from build123d import *

# Parameters (mm, degrees)
DELETE_START           = -13.5
DELETE_FACE_1_DEPTH    = 27
MOVE_FACE_1_BY         = 7
MOVE_FACE_2_BY         = 5.5
SKETCH_2_W             = 48.263019836
SKETCH_2_H             = 43.058184364
CUT_EXTRUDE_1_DEPTH    = 20
EXTRUDE_1_DEPTH        = 2
EXTRUDE_1_DEPTH_BACK   = 5
SKETCH_3_W             = 20
SKETCH_3_H             = 19
HOLE_WIZARD_M5_1_D     = 4.2
HOLE_WIZARD_M5_1_DEPTH = 20
HOLE_WIZARD_M5_1_TIP   = 1.2618073


with BuildPart() as part:
    # Delete Face 1: read off the stored shape, not the designer's step
    # Delete Face 1 outline → Delete Face 1 (new body)
    with BuildSketch(Plane.YZ.offset(DELETE_START)):
        with BuildLine():
            ThreePointArc((-8.364285714, 23.895568572), (-8.397831007, 23.931741933), (-8.41, 23.979551078))
            Line((-8.41, 23.979551078), (-8.41, 26.020448922))
            ThreePointArc((-8.41, 26.020448922), (-8.397831007, 26.068258067), (-8.364285714, 26.104431428))
            ThreePointArc((-8.364285714, 26.104431428), (-7.725958169, 26.423724028), (-7.033327746, 26.595982314))
            ThreePointArc((-7.033327746, 26.595982314), (-6.723611818, 26.762379014), (-6.6, 27.091517187))
            Line((-6.6, 27.091517187), (-6.6, 27.908482813))
            ThreePointArc((-6.6, 27.908482813), (-6.723615527, 28.237625227), (-7.033338915, 28.404019189))
            ThreePointArc((-7.033338915, 28.404019189), (-7.725963455, 28.576277924), (-8.364285714, 28.895568572))
            ThreePointArc((-8.364285714, 28.895568572), (-8.397831007, 28.931741933), (-8.41, 28.979551078))
            Line((-8.41, 28.979551078), (-8.41, 31.020448922))
            ThreePointArc((-8.41, 31.020448922), (-8.397831007, 31.068258067), (-8.364285714, 31.104431428))
            ThreePointArc((-8.364285714, 31.104431428), (-7.725958168, 31.423724029), (-7.033327744, 31.595982314))
            ThreePointArc((-7.033327744, 31.595982314), (-6.723611817, 31.762379015), (-6.6, 32.091517187))
            Line((-6.6, 32.091517187), (-6.6, 32.908482813))
            ThreePointArc((-6.6, 32.908482813), (-6.602116164, 32.954435895), (-6.608446743, 33))
            Line((-6.608446743, 33), (-12.6, 33))
            Line((-12.6, 33), (-12.6, -33))
            Line((-12.6, -33), (-6.608446743, -33))
            ThreePointArc((-6.608446743, -33), (-6.602116164, -32.954435895), (-6.6, -32.908482813))
            Line((-6.6, -32.908482813), (-6.6, -32.091517187))
            ThreePointArc((-6.6, -32.091517187), (-6.723615531, -31.762374768), (-7.033338927, -31.595980809))
            ThreePointArc((-7.033338927, -31.595980809), (-7.72596346, -31.423722074), (-8.364285714, -31.104431428))
            ThreePointArc((-8.364285714, -31.104431428), (-8.397831007, -31.068258067), (-8.41, -31.020448922))
            Line((-8.41, -31.020448922), (-8.41, -28.979551078))
            ThreePointArc((-8.41, -28.979551078), (-8.397831007, -28.931741933), (-8.364285714, -28.895568572))
            ThreePointArc((-8.364285714, -28.895568572), (-7.725958168, -28.576275971), (-7.033327744, -28.404017686))
            ThreePointArc((-7.033327744, -28.404017686), (-6.723611817, -28.237620985), (-6.6, -27.908482813))
            Line((-6.6, -27.908482813), (-6.6, -27.091517187))
            ThreePointArc((-6.6, -27.091517187), (-6.723615528, -26.762374772), (-7.033338917, -26.595980811))
            ThreePointArc((-7.033338917, -26.595980811), (-7.725963456, -26.423722076), (-8.364285714, -26.104431428))
            ThreePointArc((-8.364285714, -26.104431428), (-8.397831007, -26.068258067), (-8.41, -26.020448922))
            Line((-8.41, -26.020448922), (-8.41, -23.979551078))
            ThreePointArc((-8.41, -23.979551078), (-8.397831007, -23.931741933), (-8.364285714, -23.895568572))
            ThreePointArc((-8.364285714, -23.895568572), (-7.725958169, -23.576275972), (-7.033327746, -23.404017686))
            ThreePointArc((-7.033327746, -23.404017686), (-6.723611818, -23.237620986), (-6.6, -22.908482813))
            Line((-6.6, -22.908482813), (-6.6, -22.091517187))
            ThreePointArc((-6.6, -22.091517187), (-6.723615529, -21.76237477), (-7.033338921, -21.59598081))
            ThreePointArc((-7.033338921, -21.59598081), (-7.725963458, -21.423722075), (-8.364285714, -21.104431428))
            ThreePointArc((-8.364285714, -21.104431428), (-8.397831007, -21.068258067), (-8.41, -21.020448922))
            Line((-8.41, -21.020448922), (-8.41, -18.979551078))
            ThreePointArc((-8.41, -18.979551078), (-8.397831007, -18.931741933), (-8.364285714, -18.895568572))
            ThreePointArc((-8.364285714, -18.895568572), (-7.725958168, -18.576275971), (-7.033327744, -18.404017686))
            ThreePointArc((-7.033327744, -18.404017686), (-6.723611817, -18.237620985), (-6.6, -17.908482813))
            Line((-6.6, -17.908482813), (-6.6, -17.091517187))
            ThreePointArc((-6.6, -17.091517187), (-6.723615531, -16.762374768), (-7.033338926, -16.595980809))
            ThreePointArc((-7.033338926, -16.595980809), (-7.72596346, -16.423722074), (-8.364285714, -16.104431428))
            ThreePointArc((-8.364285714, -16.104431428), (-8.397831007, -16.068258067), (-8.41, -16.020448922))
            Line((-8.41, -16.020448922), (-8.41, -13.979551078))
            ThreePointArc((-8.41, -13.979551078), (-8.397831007, -13.931741933), (-8.364285714, -13.895568572))
            ThreePointArc((-8.364285714, -13.895568572), (-7.725958337, -13.576276034), (-7.033328102, -13.404017734))
            ThreePointArc((-7.033328102, -13.404017734), (-6.723611936, -13.237621121), (-6.6, -12.908482813))
            Line((-6.6, -12.908482813), (-6.6, -12.091517187))
            ThreePointArc((-6.6, -12.091517187), (-6.723615532, -11.762374767), (-7.033338929, -11.595980809))
            ThreePointArc((-7.033338929, -11.595980809), (-7.725963462, -11.423722074), (-8.364285714, -11.104431428))
            ThreePointArc((-8.364285714, -11.104431428), (-8.397831007, -11.068258067), (-8.41, -11.020448922))
            Line((-8.41, -11.020448922), (-8.41, -8.979551078))
            ThreePointArc((-8.41, -8.979551078), (-8.397831007, -8.931741933), (-8.364285714, -8.895568572))
            ThreePointArc((-8.364285714, -8.895568572), (-7.725958524, -8.576276103), (-7.033328496, -8.404017787))
            ThreePointArc((-7.033328496, -8.404017787), (-6.723612067, -8.23762127), (-6.6, -7.908482813))
            Line((-6.6, -7.908482813), (-6.6, -7.091517187))
            ThreePointArc((-6.6, -7.091517187), (-6.723615306, -6.762375026), (-7.033338249, -6.595980901))
            ThreePointArc((-7.033338249, -6.595980901), (-7.72596314, -6.423722193), (-8.364285714, -6.104431428))
            ThreePointArc((-8.364285714, -6.104431428), (-8.397831007, -6.068258067), (-8.41, -6.020448922))
            Line((-8.41, -6.020448922), (-8.41, -3.979551078))
            ThreePointArc((-8.41, -3.979551078), (-8.397831007, -3.931741933), (-8.364285714, -3.895568572))
            ThreePointArc((-8.364285714, -3.895568572), (-7.725958462, -3.57627608), (-7.033328366, -3.40401777))
            ThreePointArc((-7.033328366, -3.40401777), (-6.723612024, -3.237621221), (-6.6, -2.908482813))
            Line((-6.6, -2.908482813), (-6.6, -2.091517187))
            ThreePointArc((-6.6, -2.091517187), (-6.723615307, -1.762375024), (-7.033338252, -1.5959809))
            ThreePointArc((-7.033338252, -1.5959809), (-7.725963141, -1.423722192), (-8.364285714, -1.104431428))
            ThreePointArc((-8.364285714, -1.104431428), (-8.397831007, -1.068258067), (-8.41, -1.020448922))
            Line((-8.41, -1.020448922), (-8.41, 1.020448922))
            ThreePointArc((-8.41, 1.020448922), (-8.397831007, 1.068258067), (-8.364285714, 1.104431428))
            ThreePointArc((-8.364285714, 1.104431428), (-7.725958462, 1.42372392), (-7.033328366, 1.59598223))
            ThreePointArc((-7.033328366, 1.59598223), (-6.723612024, 1.762378779), (-6.6, 2.091517187))
            Line((-6.6, 2.091517187), (-6.6, 2.908482813))
            ThreePointArc((-6.6, 2.908482813), (-6.723615307, 3.237624975), (-7.033338252, 3.4040191))
            ThreePointArc((-7.033338252, 3.4040191), (-7.725963141, 3.576277808), (-8.364285714, 3.895568572))
            ThreePointArc((-8.364285714, 3.895568572), (-8.397831007, 3.931741933), (-8.41, 3.979551078))
            Line((-8.41, 3.979551078), (-8.41, 6.020448922))
            ThreePointArc((-8.41, 6.020448922), (-8.397831007, 6.068258067), (-8.364285714, 6.104431428))
            ThreePointArc((-8.364285714, 6.104431428), (-7.725958469, 6.423723918), (-7.03332838, 6.595982228))
            ThreePointArc((-7.03332838, 6.595982228), (-6.723612029, 6.762378774), (-6.6, 7.091517187))
            Line((-6.6, 7.091517187), (-6.6, 7.908482813))
            ThreePointArc((-6.6, 7.908482813), (-6.723615311, 8.23762498), (-7.033338263, 8.404019101))
            ThreePointArc((-7.033338263, 8.404019101), (-7.725963146, 8.57627781), (-8.364285714, 8.895568572))
            ThreePointArc((-8.364285714, 8.895568572), (-8.397831007, 8.931741933), (-8.41, 8.979551078))
            Line((-8.41, 8.979551078), (-8.41, 11.020448922))
            ThreePointArc((-8.41, 11.020448922), (-8.397831007, 11.068258067), (-8.364285714, 11.104431428))
            ThreePointArc((-8.364285714, 11.104431428), (-7.725958337, 11.423723966), (-7.033328101, 11.595982266))
            ThreePointArc((-7.033328101, 11.595982266), (-6.723611936, 11.76237888), (-6.6, 12.091517187))
            Line((-6.6, 12.091517187), (-6.6, 12.908482813))
            ThreePointArc((-6.6, 12.908482813), (-6.72361553, 13.237625231), (-7.033338924, 13.40401919))
            ThreePointArc((-7.033338924, 13.40401919), (-7.725963459, 13.576277925), (-8.364285714, 13.895568572))
            ThreePointArc((-8.364285714, 13.895568572), (-8.397831007, 13.931741933), (-8.41, 13.979551078))
            Line((-8.41, 13.979551078), (-8.41, 16.020448922))
            ThreePointArc((-8.41, 16.020448922), (-8.397831007, 16.068258067), (-8.364285714, 16.104431428))
            ThreePointArc((-8.364285714, 16.104431428), (-7.725958169, 16.423724029), (-7.033327745, 16.595982314))
            ThreePointArc((-7.033327745, 16.595982314), (-6.723611818, 16.762379015), (-6.6, 17.091517187))
            Line((-6.6, 17.091517187), (-6.6, 17.908482813))
            ThreePointArc((-6.6, 17.908482813), (-6.72361553, 18.23762523), (-7.033338923, 18.40401919))
            ThreePointArc((-7.033338923, 18.40401919), (-7.725963459, 18.576277925), (-8.364285714, 18.895568572))
            ThreePointArc((-8.364285714, 18.895568572), (-8.397831007, 18.931741933), (-8.41, 18.979551078))
            Line((-8.41, 18.979551078), (-8.41, 21.020448922))
            ThreePointArc((-8.41, 21.020448922), (-8.397831007, 21.068258067), (-8.364285714, 21.104431428))
            ThreePointArc((-8.364285714, 21.104431428), (-7.725958168, 21.423724029), (-7.033327744, 21.595982314))
            ThreePointArc((-7.033327744, 21.595982314), (-6.723611817, 21.762379015), (-6.6, 22.091517187))
            Line((-6.6, 22.091517187), (-6.6, 22.908482813))
            ThreePointArc((-6.6, 22.908482813), (-6.723615528, 23.237625227), (-7.033338915, 23.404019189))
            ThreePointArc((-7.033338915, 23.404019189), (-7.725963455, 23.576277924), (-8.364285714, 23.895568572))
        make_face()
    extrude(amount=DELETE_FACE_1_DEPTH)

    # Move Face 1: a face moved inward by 7.0
    extrude(part.faces().sort_by_distance((13.5, -10.05864991, 0))[0], amount=MOVE_FACE_1_BY, dir=(-1, 0, 0), mode=Mode.SUBTRACT)

    # Move Face 2: a face moved outward by 5.5
    extrude(part.faces().sort_by_distance((-3.5, -12.6, 0))[0], amount=MOVE_FACE_2_BY, dir=(0, -1, 0))

    # 草图2 → 切除-拉伸1 (cut)
    with BuildSketch(Plane.XZ.offset(18.1)):
        with Locations((-0.503276546, 28.529092182)):
            Rectangle(SKETCH_2_W, SKETCH_2_H)
    extrude(amount=-CUT_EXTRUDE_1_DEPTH, mode=Mode.SUBTRACT)

    # 草图3 → 凸台-拉伸1 (add, two sides: drawn at the far end of the back side and taken through both)
    with BuildSketch(Plane(origin=(0, -6.6, 0), x_dir=(1, 0, 0), z_dir=(0, 1, 0)).offset(-EXTRUDE_1_DEPTH_BACK)):
        with Locations((-3.5, 2.5)):
            Rectangle(SKETCH_3_W, SKETCH_3_H)
    extrude(amount=EXTRUDE_1_DEPTH + EXTRUDE_1_DEPTH_BACK)

    # M5 螺纹孔1
    with Locations(Plane(origin=(-4.186814404, -18.1, 3), x_dir=(0, 0, -1), z_dir=(0, -1, 0))):
        with Locations((0, 0), (13.5, 0)):
            Hole(HOLE_WIZARD_M5_1_D / 2, depth=HOLE_WIZARD_M5_1_DEPTH)
            with Locations((0, 0, -(HOLE_WIZARD_M5_1_DEPTH + HOLE_WIZARD_M5_1_TIP / 2))):  # 118° drill point
                Cone(0, HOLE_WIZARD_M5_1_D / 2, HOLE_WIZARD_M5_1_TIP, mode=Mode.SUBTRACT)


solid = part.part
The model under review builds one solid part; all positions refer to its coordinate system, in mm. A direction names the side the tool comes from. Round coordinates to 2 decimals unless told otherwise and drop trailing zeros. Write each loop counter-clockwise with the first axis right and the second up, starting at its lowest first coordinate (ties: lowest second). Pieces come first, ordered by that corner, then holes. Notation, with made-up numbers: M 72.25,80.25 L 120.25,80.25 A13 ccw 120.25,104.25 Z; hole C -21.5,-4.5 d7. An arc over 180 degrees is marked long. Use a Markdown table: item, result. Add a question column.
Q1. We need section A-A, the plane z = 3. State the section outline as (x, y) points.
Q2. The part is to be moulded in two halves that separate along Z. For faces 4 (the face through (-4, -8.41, -30)), 5 (the face through (-3.6, -6.6, -12.7)), 6 (the face through (2, -6, -12)), say which applies: pulls with the +Z half, pulls with the -Z half, needs draft (parallel to the pull), parting line crosses it, or undercut.
Q3. We need section C-C, the plane z = -25. State the section outline as (x, y) points, plus the area to 3 significant figures.
Q4. Insertion check: pin 1 (0.9 mm diameter, centred on x = -6, z = -27.5, fed in from +Y); pin 2 (1.6 mm diameter, centred on x = -0.5, z = -30.5, fed in from +Y); pin 3 (1 mm diameter, centred on x = -6.5, z = -20.5, fed in from +Y); pin 4 (3.5 mm diameter, centred on x = -4.19, z = -10.5, fed in from -Y). Each pin has a flat end and moves straight along its axis. Give the tip position at first contact, or say it passes through.
Q5. To check wall thickness, follow line 1 (X direction, y = -10, z = -10.5); line 2 (Z direction, x = -4.5, y = -17); line 3 (Y direction, x = -0.75, z = -29). State the ranges of each line that lie inside material, in increasing order.
Q6. Machinability: for faces 1 (the face through (-3.556, -11.256, 5.003)), 2 (the face through (-3.64, -7.74, -13.58)), 3 (the face through (-3.6, -6.6, -27.5)), which of the approach directions +Z, -Z, +X, -X, +Y, -Y give a long, thin tool a straight path to every point of the face, cutting with its end or side? Answer none if there is none.
Q7. We need section B-B, the plane y = -9.5. State the section outline as (x, z) points.
Findings below:
| question | item | result |
|---|---|---|
| 1 | outline | M -13.5,-18.1 L -6.29,-18.1 L -6.29,-4.6 L -13.5,-4.6 Z; M -2.09,-18.1 L 6.5,-18.1 L 6.5,-4.6 L -2.09,-4.6 Z |
| 2 | face 4 | undercut |
| 2 | face 5 | needs draft |
| 2 | face 6 | pulls with the -Z half |
| 3 | outline | M -13.5,-18.1 L 6.5,-18.1 L 6.5,-8.41 L -13.5,-8.41 Z |
| 3 | area | 194 mm² |
| 4 | pin 1 | stops at y = -6.6 |
| 4 | pin 2 | stops at y = -8.02 |
| 4 | pin 3 | stops at y = -8.41 |
| 4 | pin 4 | passes through |
| 5 | line 1 | x = -13.5 to -6.29, -2.09 to 6.5 |
| 5 | line 2 | z = -33 to -12.58, -8.42 to 0.92, 5.08 to 7 |
| 5 | line 3 | y = -18.1 to -8.41 |
| 6 | face 1 | +Y, -Y |
| 6 | face 2 | +X, -X, +Y |
| 6 | face 3 | -Z, +X, -X, +Y |
| 7 | outline | M -13.5,-33 L 6.5,-33 L 6.5,7 L -13.5,7 Z; hole C -4.19,-10.5 d4.2; hole C -4.19,3 d4.2 |
